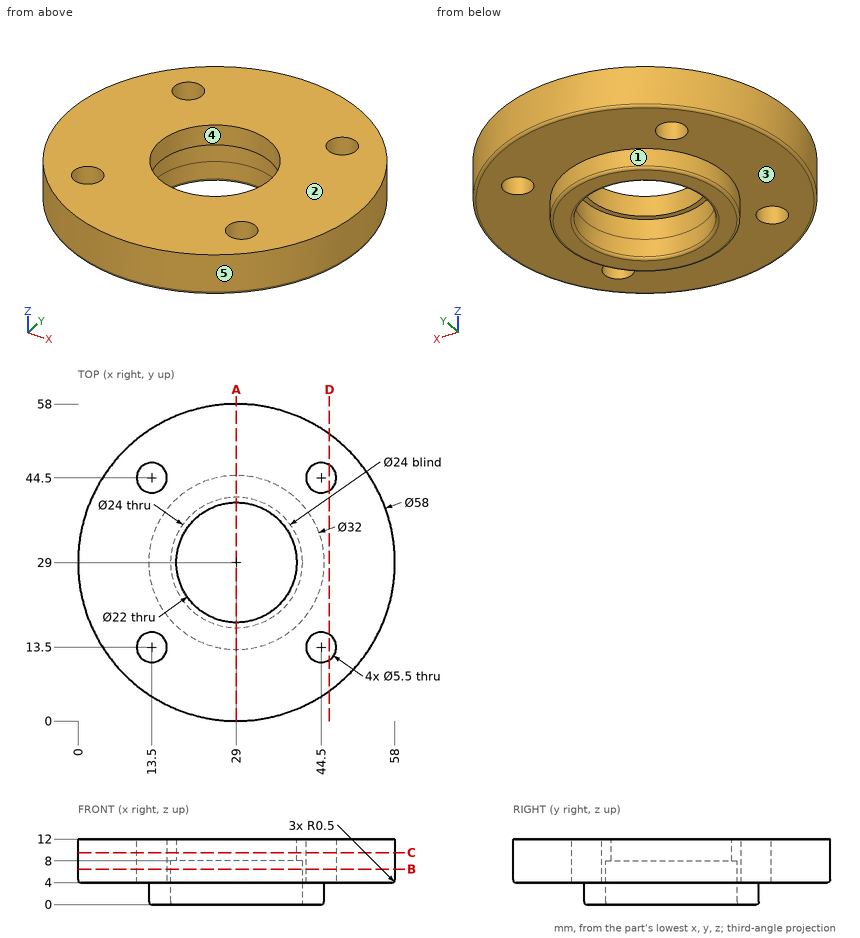
Print and shaded views of the part. All mm, measured from the part's lowest x, y and z. A direction names the side the tool comes from. Give positions to 0.01 mm unless a question says otherwise; leave off trailing zeros. Write each loop counter-clockwise with the first axis right and the second up, starting at its lowest first coordinate (ties: lowest second). Pieces come first, ordered by that corner, then holes. Notation, with made-up numbers: M 47,-29 L 84,-29 A14 ccw 84,-7 Z; hole C 3,-35.5 d4. An arc over 180 degrees is marked long. Use a Markdown table: item, result.
1) Cut at D-D (x = 46). Give the number of separate pieces and of enclosed holes in the cut face, and give its area (3 significant figures).
Responses:
| item | result |
|---|---|
| separate pieces | 3 |
| enclosed holes | 0 |
| area | 302 mm2 |
2) Cut at C-C (z = 9.5). List the corners of the cut face in (x, y), and give its area (3 significant figures).
Responses:
| item | result |
|---|---|
| outline | C 29,29 d58; hole C 13.5,13.5 d5.5; hole C 13.5,44.5 d5.5; hole C 29,29 d22; hole C 44.5,13.5 d5.5; hole C 44.5,44.5 d5.5 |
| area | 2,170 mm2 |
3) Cut at A-A (x = 29). List the corners of the cut face in (y, z), and give its area (3 significant figures).
Responses:
| item | result |
|---|---|
| outline | M 0,4.5 A0.5 ccw 0.5,4 L 13,4 L 13,0.5 A0.5 ccw 13.5,0 L 16.5,0 A0.5 ccw 17,0.5 L 17,8 L 18,8 L 18,12 L 0,12 Z; M 40,8 L 41,8 L 41,0.5 A0.5 ccw 41.5,0 L 44.5,0 A0.5 ccw 45,0.5 L 45,4 L 57.5,4 A0.5 ccw 58,4.5 L 58,12 L 40,12 Z |
| area | 312 mm2 |
4) Pull direction X, two halves, no side cores. Call the marked faces 3, 4 and 5: +X half, -X half, draft (parallel to the pull), parting line (faces both ways), or undercut.
Responses:
| item | result |
|---|---|
| face 3 | draft |
| face 4 | undercut |
| face 5 | parting line |
5) Cut at B-B (z = 6.5). List the corners of the cut face in (x, y), and give its area (3 significant figures).
Responses:
| item | result |
|---|---|
| outline | C 29,29 d58; hole C 13.5,13.5 d5.5; hole C 13.5,44.5 d5.5; hole C 29,29 d24; hole C 44.5,13.5 d5.5; hole C 44.5,44.5 d5.5 |
| area | 2,090 mm2 |
6) Tool access for the marked faces 1 and 2: list every direction of +Z, -Z, +X, -X, +Y, -Y with a clear straight run to the whole face (end or side of a thin tool).
Responses:
| item | result |
|---|---|
| face 1 | -Z |
| face 2 | +Z, +X, -X, +Y, -Y |
7) Drill centre lines: line 1 (Y direction, x = 13, z = 5); line 2 (Z direction, x = 11, y = 12); line 3 (Y direction, x = 23.5, z = 5.5). Where is each one in solid material? Low to high. Write a range as from..to.
Responses:
| item | result |
|---|---|
| line 1 | y = 4.81..10.8, 16.2..41.8, 47.2..53.19 |
| line 2 | z = 4..12 |
| line 3 | y = 0.53..18.33, 39.67..57.47 |
8) Pin check, flat tips, straight feed: pin 1 (4 mm diameter, centred on x = 46.5, z = 2.5, fed in from -Y); pin 2 (5 mm diameter, centred on x = 13.5, y = 44.5, fed in from -Z); pin 3 (1 mm diameter, centred on y = 14, z = 2, fed in from +X); pin 4 (1.5 mm diameter, centred on y = 7, z = 3.5, fed in from -X). Stop position of each tip, or through.
Responses:
| item | result |
|---|---|
| pin 1 | stops at y = 5.23 |
| pin 2 | passes through |
| pin 3 | stops at x = 35.76 |
| pin 4 | stops at x = 9.89 |
